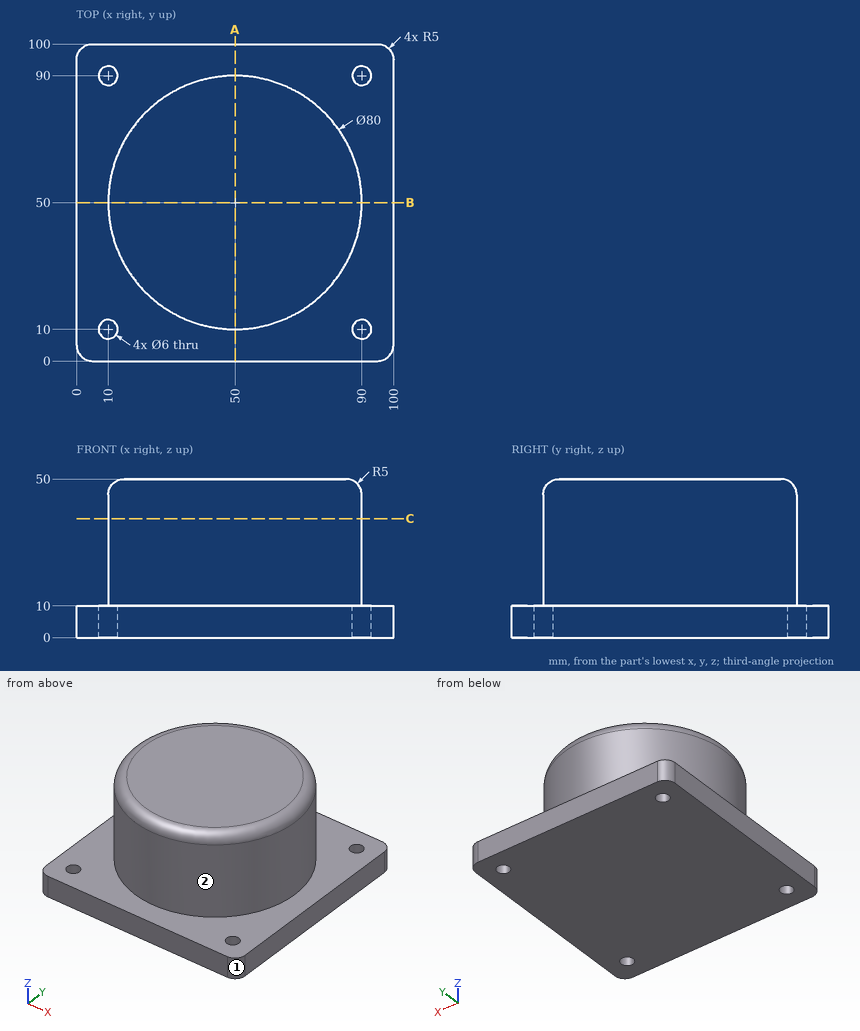
Study the drawing (mm; zero at the part's minimum x, y, z) and answer. A direction names the side the tool comes from. Coordinates: 2 decimals unless noted, no trailing zeros. Write each loop counter-clockwise with the first axis right and the second up, starting at its lowest first coordinate (ties: lowest second). Pieces come first, ordered by that corner, then holes. Notation, with made-up numbers: M 48,-8 L 67,-8 A27 ccw 67,24 Z; hole C -40,5.25 d1. An arc over 180 degrees is marked long. Use a Markdown table: item, result. Add a question column.
1. Which of the six approach directions +Z, -Z, +X, -X, +Y, -Y give full straight-line access (tool end or side, diameter ignored) to the marked faces 1 and 2?
2. Section A-A (x = 50) is taken. Give the vertices of the cut face in (y, z), plus the area to 3 significant figures.
3. Section C-C (z = 37.5) is taken. Give the vertices of the cut face in (x, y), plus the area to 3 significant figures.
4. Given P1, Ø5.5, axis at x = 10, y = 10, coming from the +Z side; P2, Ø1.5, axis at y = 79, z = 11, coming from the -X side; P3, Ø4, axis at x = 63.5, z = 15.5, coming from the +Y side; P4, Ø5, axis at y = 34.5, z = 16, coming from the -X side, each flat-ended and moving along its own axis, determine where each tip first touches the part or whether it passes through.
5. Straight lines are drawn through the part: line 1 along Y through (x, z) = (90, 8); line 2 along Z through (x, y) = (11, 64); line 3 along Y through (x, z) = (87, 44). For each, find the intervals that lie inside material, in ascending order. Write a range as [from, to].
Data:
| question | item | result |
|---|---|---|
| 1 | face 1 | +Z, -Z, +X, -Y |
| 1 | face 2 | +Z |
| 2 | outline | M 0,0 L 100,0 L 100,10 L 90,10 L 90,45 A5 ccw 85,50 L 15,50 A5 ccw 10,45 L 10,10 L 0,10 Z |
| 2 | area | 4,190 mm2 |
| 3 | outline | C 50,50 d80 |
| 3 | area | 5,030 mm2 |
| 4 | P1 | passes through |
| 4 | P2 | stops at x = 21.68 |
| 4 | P3 | stops at y = 88.31 |
| 4 | P4 | stops at x = 12.17 |
| 5 | line 1 | y = [0, 7], [13, 87], [93, 100] |
| 5 | line 2 | z = [0, 10] |
| 5 | line 3 | y = [34.8, 65.2] |
